```python
from build123d import *

# Parameters (mm, degrees)
SKETCH_1_W      = 38
SKETCH_1_H      = 38
SKETCH_1_R      = 1.3
EXTRUDE_1_DEPTH = 2
SKETCH_2_W      = 17
SKETCH_2_H      = 17
EXTRUDE_2_DEPTH = 4
SKETCH_3_R      = 8.5
EXTRUDE_3_DEPTH = 15
EXTRUDE_4_DEPTH = 4


with BuildPart() as part:
    # 草图1 → 凸台-拉伸1 (new body)
    with BuildSketch(Plane(origin=(0, 0, 0), x_dir=(1, 0, 0), z_dir=(0, 1, 0))):
        Rectangle(SKETCH_1_W, SKETCH_1_H)
        with Locations(Location((-14, -14, 0), (0, 0, 270))):
            Circle(SKETCH_1_R, mode=Mode.SUBTRACT)
        with Locations(Location((-14, 14, 0), (0, 0, 270))):
            Circle(SKETCH_1_R, mode=Mode.SUBTRACT)
        with Locations(Location((14, 14, 0), (0, 0, 270))):
            Circle(SKETCH_1_R, mode=Mode.SUBTRACT)
        with Locations(Location((14, -14, 0), (0, 0, 270))):
            Circle(SKETCH_1_R, mode=Mode.SUBTRACT)
    extrude(amount=EXTRUDE_1_DEPTH)

    # 草图2 → 凸台-拉伸2 (add)
    with BuildSketch(Plane(origin=(0, 2, 0), x_dir=(1, 0, 0), z_dir=(0, 1, 0))):
        Rectangle(SKETCH_2_W, SKETCH_2_H)
    extrude(amount=EXTRUDE_2_DEPTH)

    # 草图3 → 凸台-拉伸3 (add)
    with BuildSketch(Plane(origin=(0, 6, 0), x_dir=(1, 0, 0), z_dir=(0, 1, 0))):
        with Locations(Location((0, 0, 0), (0, 0, 270))):
            Circle(SKETCH_3_R)
    extrude(amount=EXTRUDE_3_DEPTH)

    # 草图4 → 凸台-拉伸4 (add)
    with BuildSketch(Plane(origin=(0, 2, 0), x_dir=(1, 0, 0), z_dir=(0, 1, 0))):
        with BuildLine():
            Line((-10, 2.5), (10, 2.5))
            ThreePointArc((10, 2.5), (12.5, 0), (10, -2.5))
            Line((10, -2.5), (-10, -2.5))
            ThreePointArc((-10, -2.5), (-12.5, 0), (-10, 2.5))
        make_face()
    extrude(amount=EXTRUDE_4_DEPTH)


solid = part.part
```
Can you work these out from the model? Positions are in its coordinate system, mm. A direction names the side the tool comes from. Round coordinates to 2 decimals unless told otherwise and drop trailing zeros. Loops run counter-clockwise (first coordinate to the right, second up) from the corner with the lowest first, then second, coordinate; pieces in that order, holes last. Notation, with made-up numbers: (-17.5, 41) -> (-0.5, 41) arc R17 cw to (-0.5, 54) -> close; hole circle Ø4 at (-27.5, 86.5). An arc over 180 degrees is marked (long way). Answer in a Markdown table with one row per item.
Item 1: If I drill on probe 1 along X at (y, z) = (0.55, 14); probe 2 along X at (y, z) = (3.5, -7); probe 3 along Y at (x, z) = (-12, -0.5), over which ranges is the centre line in solid material (lowest first)?
Answer block:
| item | result |
|---|---|
| probe 1 | -19 to -15.3, -12.7 to 12.7, 15.3 to 19 |
| probe 2 | -8.5 to 8.5 |
| probe 3 | 0 to 6 |
Item 2: We'd pull the mould along Z, two halves only. Please class faces 1 (the flat face through (0, 4, -8.5)), 2 (the cylindrical face through (-13.94, 0.99, 12.7)), 3 (the flat face through (-9, 4, 2.5)): released by +Z, released by -Z, zero draft, split by the parting line, or undercut.
Answer block:
| item | result |
|---|---|
| face 1 | released by -Z |
| face 2 | undercut |
| face 3 | released by +Z |
Item 3: Will these pins go through, and if not, where does the flat tip stop? P1, Ø1.5, axis at x = 4.5, y = 16, coming from the +Z side; P2, Ø3.5, axis at x = 14, z = 14, coming from the +Y side; P3, Ø12, axis at x = -0.5, y = 15, coming from the +Z side.
Answer block:
| item | result |
|---|---|
| P1 | z = 7.63 |
| P2 | y = 2 |
| P3 | z = 8.5 |
Item 4: Suppose I cut it at B-B, the plane z = 14. List the corners of the cut face in (x, y) for me, plus the area to 3 significant figures.
Answer block:
| item | result |
|---|---|
| outline | (-19, 0) -> (-15.3, 0) -> (-15.3, 2) -> (-19, 2) -> close; (-12.7, 0) -> (12.7, 0) -> (12.7, 2) -> (-12.7, 2) -> close; (15.3, 0) -> (19, 0) -> (19, 2) -> (15.3, 2) -> close |
| area | 65.6 mm² |
Item 5: Suppose I cut it at D-D, the plane y = 5.5. List the corners of the cut face in (x, z) for me, plus the area to 3 significant figures.
Answer block:
| item | result |
|---|---|
| outline | (-10, -2.5) -> (-8.5, -2.5) -> (-8.5, -8.5) -> (8.5, -8.5) -> (8.5, -2.5) -> (10, -2.5) arc R2.5 ccw to (10, 2.5) -> (8.5, 2.5) -> (8.5, 8.5) -> (-8.5, 8.5) -> (-8.5, 2.5) -> (-10, 2.5) arc R2.5 ccw to start |
| area | 324 mm² |
Item 6: Suppose I cut it at C-C, the plane z = 0. List the corners of the cut face in (x, y) for me, plus the area to 3 significant figures.
Answer block:
| item | result |
|---|---|
| outline | (-19, 0) -> (19, 0) -> (19, 2) -> (12.5, 2) -> (12.5, 6) -> (8.5, 6) -> (8.5, 21) -> (-8.5, 21) -> (-8.5, 6) -> (-12.5, 6) -> (-12.5, 2) -> (-19, 2) -> close |
| area | 431 mm² |
Item 7: Suppose I cut it at A-A, the plane x = -14. List the corners of the cut face in (y, z) for me.
Answer block:
| item | result |
|---|---|
| outline | (0, -19) -> (2, -19) -> (2, -15.3) -> (0, -15.3) -> close; (0, -12.7) -> (2, -12.7) -> (2, 12.7) -> (0, 12.7) -> close; (0, 15.3) -> (2, 15.3) -> (2, 19) -> (0, 19) -> close |
Item 8: On a 3-axis mill with a long thin cutter (end or side, diameter ignored), from which of +Z, -Z, +X, -X, +Y, -Y can I reach the whole of each face in a straight line? I mean faces 4 (the flat face through (-8.5, 4, -5)), 5 (the flat face through (-8.5, 4, 6)), 6 (the flat face through (-9, 6, 0)), 7 (the cylindrical face through (-5.172, 13.395, -6.745)). Say none if no direction works.
Answer block:
| item | result |
|---|---|
| face 4 | -Z, -X, +Y |
| face 5 | +Z, -X, +Y |
| face 6 | -X, +Y |
| face 7 | +Y |
